Design review of the part shown in the three views and the two pictorial views. Dimensions are in mm from the part's minimum x, y and z. A direction names the side the tool comes from. Give positions to 0.01 mm unless a question says otherwise; leave off trailing zeros. Order: outer loops, then holes, each group sorted by start corner. A loop starts at its lowest first (then second) coordinate and runs counter-clockwise, first axis right, second up. Notation, with made-up numbers: (34.5, -24.5) - (43.5, -24.5) arc R25 ccw to (43.5, -2.5) - close; hole circle Ø8 at (-37, 69.5). An arc over 180 degrees is marked (long way). Put each result on its own line as item: value.
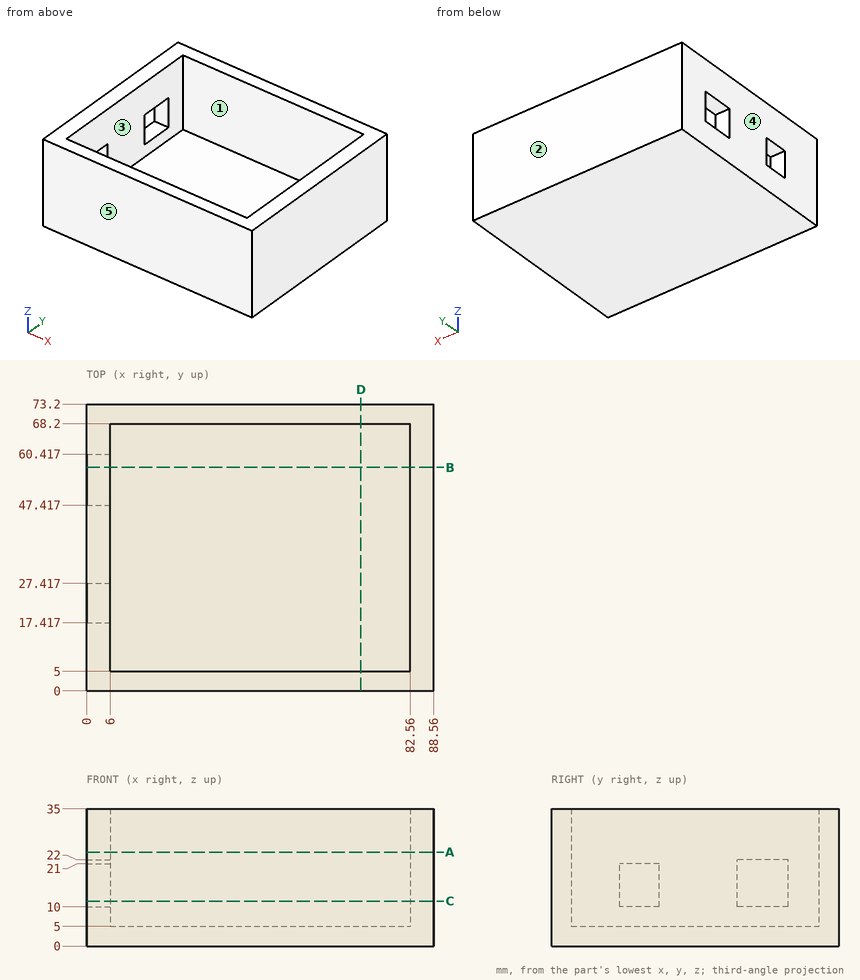
(1) Take a section at C-C, the plane z = 11.5. Write out the cut boundary in (x, y), then the cut area to 3 significant figures.
The answers:
outline: (0, 0) - (88.56, 0) - (88.56, 73.2) - (0, 73.2) - (0, 60.42) - (6, 60.42) - (6, 68.2) - (82.56, 68.2) - (82.56, 5) - (6, 5) - (6, 17.42) - (0, 17.42) - close; (0, 27.42) - (6, 27.42) - (6, 47.42) - (0, 47.42) - close
area: 1,510 mm^2
(2) Take a section at D-D, the plane x = 70. Write out the cut boundary in (y, z), then the cut area to 3 significant figures.
The answers:
outline: (0, 0) - (73.2, 0) - (73.2, 35) - (68.2, 35) - (68.2, 5) - (5, 5) - (5, 35) - (0, 35) - close
area: 666 mm^2
(3) Take a section at B-B, the plane y = 57. Write out the cut boundary in (x, z).
The answers:
outline: (0, 0) - (88.56, 0) - (88.56, 35) - (82.56, 35) - (82.56, 5) - (6, 5) - (6, 10) - (0, 10) - close; (0, 22) - (6, 22) - (6, 35) - (0, 35) - close
(4) Wall thickness on L1, parallel to X at y = 35.5, z = 22; L2, parallel to Y at x = 59, z = 12.5; L3, parallel to X at y = 47.5, z = 12: over which ranges is each line inside the solid? List them lowest first.
The answers:
L1: 0 to 6, 82.56 to 88.56
L2: 0 to 5, 68.2 to 73.2
L3: 82.56 to 88.56
(5) For the marked faces 1 and 2, list the 3-axis set-ups (+Z, -Z, +X, -X, +Y, -Y) from which the entire face can be reached by the end or side of a thin tool; tool diameter is ignored.
The answers:
face 1: +Z
face 2: +Z, -Z, +X, -X, +Y
(6) Take a section at A-A, the plane z = 24. Write out the cut boundary in (x, y).
The answers:
outline: (0, 0) - (88.56, 0) - (88.56, 73.2) - (0, 73.2) - close; hole (6, 5) - (82.56, 5) - (82.56, 68.2) - (6, 68.2) - close
(7) Clearance check with a flat-ended pin moving along its axis: pin 1 Ø5 at (x, y) = (30, 47.5) entering from +Z. State where the tip first meets the part, or that it passes through.
The answers:
pin 1: z = 5
(8) The part is to be moulded in two halves that separate along X. For the marked faces 3, 4 and 5, say which applies: pulls with the +X half, pulls with the -X half, needs draft (parallel to the pull), parting line crosses it, or undercut.
The answers:
face 3: undercut
face 4: pulls with the -X half
face 5: needs draft
